Here's how the part is built. I have some questions about the finished solid (model axes, mm). A direction names the side the tool comes from. Give positions to 0.01 mm unless a question says otherwise; leave off trailing zeros. Loops run counter-clockwise (first coordinate to the right, second up) from the corner with the lowest first, then second, coordinate; pieces in that order, holes last.
Q1. If we section it at B-B (y = 0): Please give me the cut outline in (x, z).
Q2. For faces 1 (the face through (-1, 14, 0)), 2 (the face through (67.57, -4, 2.28)), which set-ups out of +Z, -Z, +X, -X, +Y, -Y let a thin tool reach every point of the face, with its end or its side?
Q3. We'd pull the mould along X, two halves only. Please class faces 3 (the face through (36, -47.5, 2)), 4 (the face through (67.5, -46.07, 2.28)), 5 (the face through (-77.57, -56, 2.28)), 6 (the face through (-1, -57.5, 2)): +X half, -X half, draft (parallel to the pull), parting line (faces both ways), or undercut.
Q4. I need wall thicknesses on line 1 (X direction, y = -34, z = 1.85); line 2 (Y direction, x = -72, z = 2.2); line 3 (X direction, y = -51.5, z = 1.65). Which ranges of each line are inside material? Lowest first, please.
Q5. Will this pin go through, and if not, where does the flat tip stop? P1, Ø4.5, axis at x = -72, y = 50.5, coming from the +Z side.
Q6. If we section it at C-C (y = -50.5): Please give me the cut outline in (x, z), plus the area to 3 significant figures.
Q7. If we section it at D-D (z = 3.4): Give the number of separate pieces and of enclosed holes in the cut face, plus the area to 3 significant figures.
Q8. If we section it at A-A (x = 0): Please give me the cut outline in (y, z), plus the area to 3 significant figures.
from build123d import *

# Parameters (mm, degrees)
SKETCH_1_W          = 158
SKETCH_1_H          = 115
EXTRUDE_1_DEPTH     = 4.5
SKETCH_2_R          = 2.6
SKETCH_2_R_2        = 1.6
CUT_EXTRUDE_1_DEPTH = 4.5
FILLET_1_R          = 5


with BuildPart() as part:
    # 草图1 → 凸台-拉伸1 (new body)
    with BuildSketch(Plane.XY):
        Rectangle(SKETCH_1_W, SKETCH_1_H)
    extrude(amount=EXTRUDE_1_DEPTH)

    # 草图2 → 切除-拉伸1 (cut)
    with BuildSketch(Plane.XY.offset(4.5)):
        with Locations((-72, 50.5)):
            Circle(SKETCH_2_R)
        with Locations((72, 50.5)):
            Circle(SKETCH_2_R)
        with Locations((72, 0)):
            Circle(SKETCH_2_R)
        with Locations((72, -50.5)):
            Circle(SKETCH_2_R)
        with Locations((-72, -50.5)):
            Circle(SKETCH_2_R)
        with Locations((-72, 0)):
            Circle(SKETCH_2_R)
        Circle(SKETCH_2_R_2)
        with BuildLine():
            Line((4, -7.5), (4, -42.5))
            ThreePointArc((4, -42.5), (5.464466094, -46.035533906), (9, -47.5))
            Line((9, -47.5), (64, -47.5))
            ThreePointArc((64, -47.5), (67.535533906, -46.035533906), (69, -42.5))
            Line((69, -42.5), (69, -7.5))
            ThreePointArc((69, -7.5), (67.535533906, -3.964466094), (64, -2.5))
            Line((64, -2.5), (9, -2.5))
            ThreePointArc((9, -2.5), (5.464466094, -3.964466094), (4, -7.5))
        make_face()
        with BuildLine():
            Line((-64, -2.5), (-9, -2.5))
            ThreePointArc((-9, -2.5), (-5.464466094, -3.964466094), (-4, -7.5))
            Line((-4, -7.5), (-4, -42.5))
            ThreePointArc((-4, -42.5), (-5.464466094, -46.035533906), (-9, -47.5))
            Line((-9, -47.5), (-64, -47.5))
            ThreePointArc((-64, -47.5), (-67.535533906, -46.035533906), (-69, -42.5))
            Line((-69, -42.5), (-69, -7.5))
            ThreePointArc((-69, -7.5), (-67.535533906, -3.964466094), (-64, -2.5))
        make_face()
    extrude(amount=-CUT_EXTRUDE_1_DEPTH, mode=Mode.SUBTRACT)

    # 圆角1
    fillet_1_edges = [part.edges().sort_by_distance(p)[0] for p in [
        (-79, 57.5, 2.25),
        (79, 57.5, 2.25),
        (79, -57.5, 2.25),
        (-79, -57.5, 2.25),
    ]]
    fillet(fillet_1_edges, radius=FILLET_1_R)


solid = part.part
Check sheet entries:
1. outline: (-79, 0) - (-74.6, 0) - (-74.6, 4.5) - (-79, 4.5) - close; (-69.4, 0) - (-1.6, 0) - (-1.6, 4.5) - (-69.4, 4.5) - close; (1.6, 0) - (69.4, 0) - (69.4, 4.5) - (1.6, 4.5) - close; (74.6, 0) - (79, 0) - (79, 4.5) - (74.6, 4.5) - close
2. face 1: -Z, +X, -X, +Y, -Y
2. face 2: +Z, -Z
3. face 3: undercut
3. face 4: undercut
3. face 5: -X half
3. face 6: draft
4. line 1: x = -79 to -69, -4 to 4, 69 to 79
4. line 2: y = -57.5 to -53.1, -47.9 to -2.6, 2.6 to 47.9, 53.1 to 57.5
4. line 3: x = -79 to -74.4, -69.6 to 69.6, 74.4 to 79
5. P1: passes through
6. outline: (-79, 0) - (-74.6, 0) - (-74.6, 4.5) - (-79, 4.5) - close; (-69.4, 0) - (69.4, 0) - (69.4, 4.5) - (-69.4, 4.5) - close; (74.6, 0) - (79, 0) - (79, 4.5) - (74.6, 4.5) - close
6. area: 664 mm2
7. separate pieces: 1
7. enclosed holes: 9
7. area: 12,200 mm2
8. outline: (-57.5, 0) - (-1.6, 0) - (-1.6, 4.5) - (-57.5, 4.5) - close; (1.6, 0) - (57.5, 0) - (57.5, 4.5) - (1.6, 4.5) - close
8. area: 503 mm2
